from build123d import *

# Parameters (mm, degrees)
SKETCH1_W           = 200
SKETCH1_H           = 90
BOSS_EXTRUDE1_DEPTH = 25
SKETCH2_R           = 9
CUT_EXTRUDE1_DEPTH  = 10
SKETCH2_4_R         = 11
SKETCH2_4_R_2       = 9
CUT_EXTRUDE2_DEPTH  = 7
SKETCH3_R           = 5
CUT_EXTRUDE3_DEPTH  = 15
SKETCH4_R           = 5
CUT_EXTRUDE4_DEPTH  = 15


with BuildPart() as part:
    # Sketch1 → Boss-Extrude1 (new, symmetric)
    with BuildSketch(Plane.XY):
        Rectangle(SKETCH1_W, SKETCH1_H)
    extrude(amount=BOSS_EXTRUDE1_DEPTH, both=True)

    # Sketch2 → Cut-Extrude1 (cut)
    with BuildSketch(Plane.XY.offset(25)):
        with Locations((0, 24)):
            Circle(SKETCH2_R)
    extrude(amount=-CUT_EXTRUDE1_DEPTH, mode=Mode.SUBTRACT)

    # Sketch2<4> → Cut-Extrude2 (cut)
    with BuildSketch(Plane.XY.offset(25)):
        with Locations((0, 24)):
            Circle(SKETCH2_4_R)
        with Locations((0, 24)):
            Circle(SKETCH2_4_R_2, mode=Mode.SUBTRACT)
    extrude(amount=-CUT_EXTRUDE2_DEPTH, mode=Mode.SUBTRACT)

    # Sketch3 → Cut-Extrude3 (cut)
    with BuildSketch(Plane.XZ.offset(45)):
        with Locations((-50, 0)):
            Circle(SKETCH3_R)
        with Locations((50, 0)):
            Circle(SKETCH3_R)
    extrude(amount=-CUT_EXTRUDE3_DEPTH, mode=Mode.SUBTRACT)

    # Sketch4 → Cut-Extrude4 (cut)
    with BuildSketch(Plane(origin=(0, 0, -25), x_dir=(-1, 0, 0), z_dir=(0, 0, -1))):
        with Locations((-50, -5)):
            Circle(SKETCH4_R)
        with Locations((50, -5)):
            Circle(SKETCH4_R)
    extrude(amount=-CUT_EXTRUDE4_DEPTH, mode=Mode.SUBTRACT)


solid = part.part
Verification items for the finished model (mm, model axes). A direction names the side the tool comes from. Coordinates: 2 decimals unless noted, no trailing zeros. Order: outer loops, then holes, each group sorted by start corner. A loop starts at its lowest first (then second) coordinate and runs counter-clockwise, first axis right, second up. Notation, with made-up numbers: (-31, 10.25) -> (-22, 10.25) arc R12 cw to (-22, 31.25) -> close; hole circle Ø5 at (-22.75, 88). An arc over 180 degrees is marked (long way). Put each result on its own line as item: value. Start each with the question number.
1. Cross-section at D-D, the plane y = -37. Record the boundary of the cut face in (x, z).
2. Cross-section at B-B, the plane y = 24. Record the boundary of the cut face in (x, z).
3. Material ranges on L1, parallel to Z at x = 50, y = -40.5; L2, parallel to X at y = -2, z = -20; L3, parallel to X at y = -3, z = -22, recorded low to high. Write a range as [from, to].
4. Mould release check, pull along Y, two halves, no side actions. Record for faces 1 (the flat face through (-50, -30, 0)), 2 (the flat face through (-1, 45, 0)), 3 (the cylindrical face through (-45, -5, -18)), 4 (the flat face through (-50, -5, -10)): released by +Y, released by -Y, zero draft, split by the parting line, or undercut.
5. Access from +Z, -Z, +X, -X, +Y, -Y to the whole of each face (thin tool, end or side, straight path). Record for faces 5 (the flat face through (-1, -45, 0)), 6 (the flat face through (100, -1, 0)), 7 (the cylindrical face through (55, -5, -18)), 8 (the flat face through (50, -30, 0)), 9 (the cylindrical face through (4.84, 31.59, 16.52)).
6. Go/stop test with flat-tipped pins: pin 1 Ø3 at (x, z) = (48, -0.5) entering from -Y; pin 2 Ø20.5 at (x, y) = (0, 24) entering from +Z; pin 3 Ø3 at (x, y) = (-52.5, -3) entering from -Z. Record where each tip stops, or that it passes through.
7. Cross-section at C-C, the plane z = 22. Record the boundary of the cut face in (x, y).
8. Cross-section at A-A, the plane x = 0. Record the boundary of the cut face in (y, z).
Computed:
1. outline: (-100, -25) -> (100, -25) -> (100, 25) -> (-100, 25) -> close; hole circle Ø10 at (-50, 0); hole circle Ø10 at (50, 0)
2. outline: (-100, -25) -> (100, -25) -> (100, 25) -> (11, 25) -> (11, 18) -> (9, 18) -> (9, 15) -> (-9, 15) -> (-9, 18) -> (-11, 18) -> (-11, 25) -> (-100, 25) -> close
3. L1: [-25, -5], [5, 25]
3. L2: [-100, -54], [-46, 46], [54, 100]
3. L3: [-100, -54.58], [-45.42, 45.42], [54.58, 100]
4. face 1: released by -Y
4. face 2: released by +Y
4. face 3: undercut
4. face 4: undercut
5. face 5: +Z, -Z, +X, -X, -Y
5. face 6: +Z, -Z, +X, +Y, -Y
5. face 7: -Z
5. face 8: -Y
5. face 9: +Z
6. pin 1: y = -30
6. pin 2: z = 18
6. pin 3: z = -10
7. outline: (-100, -45) -> (100, -45) -> (100, 45) -> (-100, 45) -> close; hole circle Ø22 at (0, 24)
8. outline: (-45, -25) -> (45, -25) -> (45, 25) -> (35, 25) -> (35, 18) -> (33, 18) -> (33, 15) -> (15, 15) -> (15, 18) -> (13, 18) -> (13, 25) -> (-45, 25) -> close
